```python
from build123d import *

# Parameters (mm, degrees)
BOSS_EXTRUDE1_DEPTH = 6.35
FILLET1_R           = 2
SKETCH2_R           = 4
CUT_EXTRUDE1_DEPTH  = 53.532323383


with BuildPart() as part:
    # Sketch1 → Boss-Extrude1 (new body)
    with BuildSketch(Plane(origin=(0, 0, 0), x_dir=(0, 0, -1), z_dir=(1, 0, 0))):
        Polygon((0, 40), (0, 45), (20, 45), (20, 40), (26.35, 40), (26.35, 25), (20, 25), (20, 20), (26.35, 20), (26.35, 5), (20, 5), (20, 0), (0, 0), (0, 5), (-6.35, 5), (-6.35, 20), (0, 20), (0, 25), (-6.35, 25), (-6.35, 40), align=None)
    extrude(amount=BOSS_EXTRUDE1_DEPTH)

    # Fillet1
    fillet1_edges = [part.edges().sort_by_distance(p)[0] for p in [
        (3.175, 5, 6.35),
        (3.175, 20, 6.35),
        (3.175, 25, 6.35),
        (3.175, 40, 6.35),
        (3.175, 40, -26.35),
        (3.175, 25, -26.35),
        (3.175, 20, -26.35),
        (3.175, 5, -26.35),
    ]]
    fillet(fillet1_edges, radius=FILLET1_R)

    # Sketch2 → Cut-Extrude1 (cut, through all)
    with BuildSketch(Plane(origin=(6.35, 0, 0), x_dir=(0, 0, -1), z_dir=(1, 0, 0))):
        with Locations((10, 35)):
            Circle(SKETCH2_R)
    extrude(amount=-CUT_EXTRUDE1_DEPTH, mode=Mode.SUBTRACT)


solid = part.part
```
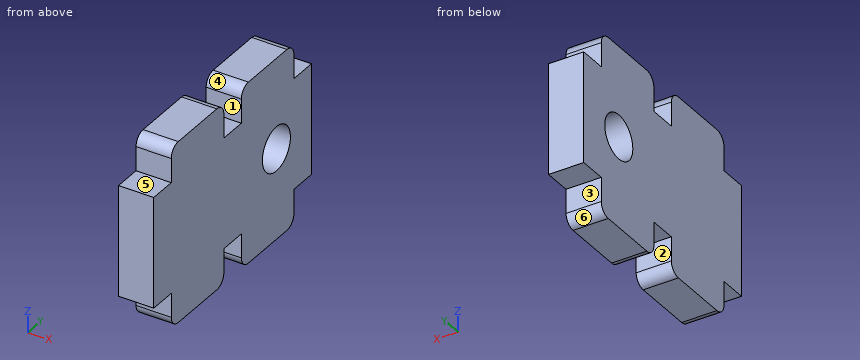
The model under review builds one solid part; all positions refer to its coordinate system, in mm. Face numbers are marked on the shaded views. A direction names the side the tool comes from. Round coordinates to 2 decimals unless told otherwise and drop trailing zeros. Order: outer loops, then holes, each group sorted by start corner. A loop starts at its lowest first (then second) coordinate and runs counter-clockwise, first axis right, second up. Notation, with made-up numbers: (52, -30) -> (57, -30) arc R25 cw to (57, -10) -> close; hole circle Ø6 at (-31, 2). An arc over 180 degrees is marked (long way). One line per item, written item: value. Start each with the question number.
Q1. Wall thickness on line 1 (Y direction, x = 2.5, z = -10); line 2 (Y direction, x = 3.5, z = 1); line 3 (Z direction, x = 0.5, y = 41): over which ranges is each line inside the solid? List them lowest first.
Q2. Take a section at A-A (y = 35). Write out the cut boundary in (x, z).
Q3. Mouldability with a two-part tool opening along Y and no side actions: class the marked faces 4, 5 and 6 as released by +Y, released by -Y, zero draft, split by the parting line, or undercut.
Q4. Take a section at B-B (z = 3). Write out the cut boundary in (x, y).
Q5. Machinability: for the marked faces 1, 2 and 3, which of the approach directions +Z, -Z, +X, -X, +Y, -Y give a long, thin tool a straight path to every point of the face, cutting with its end or side? Answer none if there is none.
Q6. Clearance check with flat-ended pins moving along their axes: pin 1 Ø3.5 at (x, z) = (2, 2) entering from -Y; pin 2 Ø3.5 at (x, z) = (3, 3) entering from +Y; pin 3 Ø3 at (x, y) = (4, 23) entering from +Z. State where each tip first meets the part, or that it passes through.
Reported:
1. line 1: y = 0 to 31, 39 to 45
1. line 2: y = 5 to 20, 25 to 40
1. line 3: z = -20 to 0
2. outline: (0, -26.35) -> (6.35, -26.35) -> (6.35, -14) -> (0, -14) -> close; (0, -6) -> (6.35, -6) -> (6.35, 6.35) -> (0, 6.35) -> close
3. face 4: undercut
3. face 5: zero draft
3. face 6: released by +Y
4. outline: (0, 5) -> (6.35, 5) -> (6.35, 20) -> (0, 20) -> close; (0, 25) -> (6.35, 25) -> (6.35, 40) -> (0, 40) -> close
5. face 1: +Z, +X, -X
5. face 2: -Z, +X, -X
5. face 3: -Z, +X, -X, +Y
6. pin 1: stops at y = 5
6. pin 2: stops at y = 40
6. pin 3: stops at z = 0
